Build history of the part. All positions in model axes, mm. A direction names the side the tool comes from. Round coordinates to 2 decimals unless told otherwise and drop trailing zeros. Write each loop counter-clockwise with the first axis right and the second up, starting at its lowest first coordinate (ties: lowest second). Pieces come first, ordered by that corner, then holes. Notation, with made-up numbers: (58.25, 70) - (73.25, 70) arc R29 ccw to (73.25, 98) - close; hole circle Ø6 at (88.5, -38). An arc over 180 degrees is marked (long way). Answer as a JSON object with one key per item and string values. Group by question number.
Item 1: Slice it at D-D, the plane x = -1.7. List the corners of the cut face in (y, z), then the cut area to 3 significant figures.
Item 2: Probe line 1 (X direction, y = 0, z = 7.8); line 2 (Y direction, x = 1.1, z = 9); line 3 (Y direction, x = 0.4, z = -4.75). List the from-to ranges inside material, lowest first. Write a range as from..to.
Item 3: Slice it at C-C, the plane y = 2.05. List the corners of the cut face in (x, z).
Item 4: Slice it at B-B, the plane z = 3.75. List the corners of the cut face in (x, y), then the cut area to 3 significant figures.
Item 5: Slice it at A-A, the plane z = -4.5. List the corners of the cut face in (x, y).
Item 6: Which spindle directions (+Z, -Z, +X, -X, +Y, -Y) get a long thin tool onto all of the face, cutting with end or side? Do faces 4 (the flat face through (-1, -1, -10)), 5 (the cylindrical face through (0.27, -1.22, 7.46)), 6 (the cylindrical face through (0.27, -1.22, -7.46)). Say none if no direction does.
Item 7: Flat gauge pins, fed straight in: pin 1 (1.5 mm diameter, centred on x = 0, y = 0, fed in from +Z); pin 2 (2 mm diameter, centred on x = 0, y = 0, fed in from -Z); pin 3 (1 mm diameter, centred on x = -0.5, y = -0.5, fed in from -Z). Where does each tip first touch, or does it go through?
Item 8: Two-plate mould, pull along Y, no slides. Class faces 1 (the flat face through (1.07, -1.88, 0.14)), 2 (the conical face through (-0.05, -0.21, 4.38)), 3 (the flat face through (-1, -1, 10)): +Y half, -Y half, draft (parallel to the pull), parting line (faces both ways), or undercut.
from build123d import *

# Parameters (mm, degrees)
F1_DEPTH = 10
F3_D     = 2.5
F3_DEPTH = 5
F3_TIP   = 0.7510757738


with BuildPart() as f1:
    # F0 (on Top) → F1 (new body)
    with BuildSketch(Plane.XY):
        Polygon((0, -2.5), (0, 0), (0, 2.5), (-2.1650635095, 1.25), (-2.1650635095, -1.25), align=None)
        Polygon((0, 2.5), (0, 0), (0, -2.5), (2.1650635095, -1.25), (2.1650635095, 1.25), align=None)
    extrude(amount=F1_DEPTH)

    # F3
    with Locations(Plane.XY.offset(10)):
        with Locations((0, 0)):
            Hole(F3_D / 2, depth=F3_DEPTH)
            with Locations((0, 0, -(F3_DEPTH + F3_TIP / 2))):  # 118° drill point
                Cone(0, F3_D / 2, F3_TIP, mode=Mode.SUBTRACT)

    # F4: F1 across plane


with BuildPart() as f1_1:
    add(f1.part)
    add(f1.part.mirror(Plane.XY))


solid = f1_1.part
Geometry says:
{
 "1": {"outline": "(-1.52, -10) - (1.52, -10) - (1.52, 10) - (-1.52, 10) - close", "area": "60.7 mm^2"},
 "2": {"line 1": "x = -2.17..-1.25, 1.25..2.17", "line 2": "y = -1.86..-0.59, 0.59..1.86", "line 3": "y = -2.27..-0.73, 0.73..2.27"},
 "3": {"outline": "(-0.78, -10) - (0.78, -10) - (0.78, 10) - (-0.78, 10) - close"},
 "4": {"outline": "(-2.17, -1.25) - (0, -2.5) - (2.17, -1.25) - (2.17, 1.25) - (0, 2.5) - (-2.17, 1.25) - close", "area": "16.2 mm^2"},
 "5": {"outline": "(-2.17, -1.25) - (0, -2.5) - (2.17, -1.25) - (2.17, 1.25) - (0, 2.5) - (-2.17, 1.25) - close; hole circle Ø0.84 at (0, 0)"},
 "6": {"face 4": "-Z, +X, -X, +Y, -Y", "face 5": "+Z", "face 6": "-Z"},
 "7": {"pin 1": "stops at z = 4.7", "pin 2": "stops at z = -4.85", "pin 3": "stops at z = -4.97"},
 "8": {"face 1": "-Y half", "face 2": "undercut", "face 3": "draft"}
}
